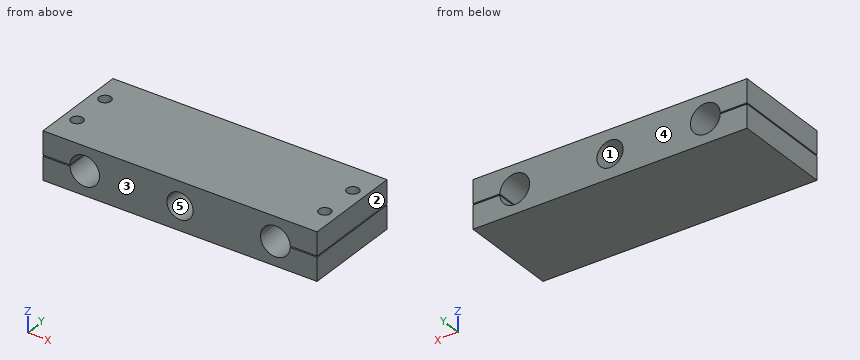
```python
from build123d import *

# Parameters (mm, degrees)
F0_W            = 230
F0_H            = 40
F1_DEPTH        = 83.5
F3_DEPTH        = 83.501
F4_R            = 11
F5_DEPTH        = 25
F6_R            = 11
F7_DEPTH        = 25
F8_W            = 26.2972414494
F8_H            = 0.5
F8_W_2          = 31.4752864838
F9_DEPTH        = 83.501
F11_D           = 8.8
F11_DEPTH       = 30
F11_CBORE_D     = 10
F11_CBORE_DEPTH = 20
F11_TIP         = 2.6437867237


with BuildPart() as f1:
    # F0 (on Front) → F1 (new body)
    with BuildSketch(Plane.XZ):
        with Locations((115, 20)):
            Rectangle(F0_W, F0_H)
    extrude(amount=F1_DEPTH)

    # F2 (on face) → F3 (cut, through all)
    with BuildSketch(Plane.XZ.offset(83.5)):
        with BuildLine():
            Line((22.5, 20), (35, 20))
            Line((35, 20), (47.5, 20))
            ThreePointArc((47.5, 20), (35, 32.5), (22.5, 20))
        make_face()
        with BuildLine():
            Line((47.5, 20), (35, 20))
            Line((35, 20), (22.5, 20))
            ThreePointArc((22.5, 20), (35, 7.5), (47.5, 20))
        make_face()
        with BuildLine():
            ThreePointArc((207.5, 20), (195, 32.5), (182.5, 20))
            Line((182.5, 20), (195, 20))
            Line((195, 20), (207.5, 20))
        make_face()
        with BuildLine():
            Line((195, 20), (182.5, 20))
            ThreePointArc((182.5, 20), (195, 7.5), (207.5, 20))
            Line((207.5, 20), (195, 20))
        make_face()
        with BuildLine():
            ThreePointArc((115, 28.5), (108.9895923599, 26.0104076401), (106.5, 20))
            Line((106.5, 20), (115, 20))
            Line((115, 20), (115, 28.5))
        make_face()
        with BuildLine():
            Line((115, 20), (106.5, 20))
            ThreePointArc((106.5, 20), (108.9895923599, 13.9895923599), (115, 11.5))
            Line((115, 11.5), (115, 20))
        make_face()
        with BuildLine():
            Line((115, 28.5), (115, 20))
            Line((115, 20), (123.5, 20))
            ThreePointArc((123.5, 20), (121.0104076401, 26.0104076401), (115, 28.5))
        make_face()
        with BuildLine():
            Line((123.5, 20), (115, 20))
            Line((115, 20), (115, 11.5))
            ThreePointArc((115, 11.5), (121.0104076401, 13.9895923599), (123.5, 20))
        make_face()
    extrude(amount=-F3_DEPTH, mode=Mode.SUBTRACT)

    # F4 (on face) → F5 (cut)
    with BuildSketch(Plane.XZ.offset(83.5)):
        with Locations((115, 20)):
            Circle(F4_R)
    extrude(amount=-F5_DEPTH, mode=Mode.SUBTRACT)

    # F6 (on face) → F7 (cut)
    with BuildSketch(Plane(origin=(0, 0, 0), x_dir=(-1, 0, 0), z_dir=(0, 1, 0))):
        with Locations((-115, 20)):
            Circle(F6_R)
    extrude(amount=-F7_DEPTH, mode=Mode.SUBTRACT)

    # F8 (on face) → F9 (cut, through all)
    with BuildSketch(Plane.XZ.offset(83.5)):
        with Locations((13.1486207247, 20.25)):
            Rectangle(F8_W, F8_H)
        with Locations((13.1486207247, 19.75)):
            Rectangle(F8_W, F8_H)
        with Locations((214.2623567581, 19.75)):
            Rectangle(F8_W_2, F8_H)
        with Locations((214.2623567581, 20.25)):
            Rectangle(F8_W_2, F8_H)
    extrude(amount=-F9_DEPTH, mode=Mode.SUBTRACT)

    # F11
    with Locations(Plane.XY.offset(40)):
        with Locations((11, -25), (11, -58.5), (219, -25), (219, -58.5)):
            CounterBoreHole(F11_D / 2, F11_CBORE_D / 2, F11_CBORE_DEPTH, depth=F11_DEPTH)
            with Locations((0, 0, -(F11_DEPTH + F11_TIP / 2))):  # 118° drill point
                Cone(0, F11_D / 2, F11_TIP, mode=Mode.SUBTRACT)


solid = f1.part
```
Here's how the part is built. I have some questions about the finished solid (model axes, mm). Face numbers are marked on the shaded views. A direction names the side the tool comes from. Round coordinates to 2 decimals unless told otherwise and drop trailing zeros. Write each loop counter-clockwise with the first axis right and the second up, starting at its lowest first coordinate (ties: lowest second). Pieces come first, ordered by that corner, then holes.
Q1. If we section it at C-C on x = 212: Write out the boundary of the cut face in (y, z).
Q2. If we mould it in two halves opening along X, with no side actions, what happens to the marked faces 1, 2 and 3? For each: +X half, -X half, draft (parallel to the pull), parting line (faces both ways), or undercut.
Q3. If we section it at B-B on y = -51.5: Write out the boundary of the cut face in (x, z).
Q4. Please list where these lines run through material, in increasing order: probe 1 along Y at (x, z) = (219, 14.25); probe 2 along X at (y, z) = (-65, 21); probe 3 along Y at (x, z) = (219, 34).
Q5. If we section it at A-A on z = 23: Write out the boundary of the cut face in (x, y), plus the area to 3 significant figures.
Q6. Will these pins go through, and if not, where does the flat tip stop? P1, Ø20, axis at x = 115, z = 20, coming from the +Y side; P2, Ø5, axis at x = 186, z = 18, coming from the -Y side.
Q7. Which directions (+Z, -Z, +X, -X, +Y, -Y) give clear straight access to the entire face, cutting with the end or side of a thin tool? Please do the marked faces 4 and 5.
Q8. If we section it at D-D on x = 189: Write out the boundary of the cut face in (y, z), plus the area to 3 significant figures.
Answer below:
1. outline: (-83.5, 0) - (0, 0) - (0, 19.5) - (-83.5, 19.5) - close; (-83.5, 20.5) - (0, 20.5) - (0, 40) - (-83.5, 40) - close
2. face 1: undercut
2. face 2: +X half
2. face 3: draft
3. outline: (0, 0) - (230, 0) - (230, 19.5) - (207.49, 19.5) arc R12.5 cw (long way) to (207.49, 20.5) - (230, 20.5) - (230, 40) - (0, 40) - (0, 20.5) - (22.51, 20.5) arc R12.5 cw (long way) to (22.51, 19.5) - (0, 19.5) - close; hole circle Ø17 at (115, 20)
4. probe 1: y = -83.5 to -62.9, -54.1 to -29.4, -20.6 to 0
4. probe 2: x = 0 to 22.54, 47.46 to 104.05, 125.95 to 182.54, 207.46 to 230
4. probe 3: y = -83.5 to -63.5, -53.5 to -30, -20 to 0
5. outline: (0, -83.5) - (22.87, -83.5) - (22.87, 0) - (0, 0) - close; (47.13, -83.5) - (104.42, -83.5) - (104.42, -58.5) - (107.05, -58.5) - (107.05, -25) - (104.42, -25) - (104.42, 0) - (47.13, 0) - close; (122.95, -58.5) - (125.58, -58.5) - (125.58, -83.5) - (182.87, -83.5) - (182.87, 0) - (125.58, 0) - (125.58, -25) - (122.95, -25) - close; (207.13, -83.5) - (230, -83.5) - (230, 0) - (207.13, 0) - close; hole circle Ø10 at (11, -58.5); hole circle Ø10 at (11, -25); hole circle Ø10 at (219, -58.5); hole circle Ø10 at (219, -25)
5. area: 13,200 mm2
6. P1: stops at y = -25
6. P2: passes through
7. face 4: +Z, -Z, +X, -X, +Y
7. face 5: -Y
8. outline: (-83.5, 0) - (0, 0) - (0, 9.03) - (-83.5, 9.03) - close; (-83.5, 30.97) - (0, 30.97) - (0, 40) - (-83.5, 40) - close
8. area: 1,510 mm2
